Can you work these out from the model? Positions are in its coordinate system, mm. Face numbers are marked on the shaded views. Coordinates: 2 decimals unless noted, no trailing zeros. Loops run counter-clockwise (first coordinate to the right, second up) from the corner with the lowest first, then second, coordinate; pieces in that order, holes last.
```python
from build123d import *

# Parameters (mm, degrees)
F0_W        = 41.65
F0_H        = 46.1
F1_DEPTH    = 6.5
F2_W        = 28.5
F2_H        = 3
F3_DEPTH    = 3
F4_R        = 1
F5_T1_DEPTH = 10.5
F5_T4_ANGLE = 90
F5_T6_ANGLE = 90
F6_W        = 20
F6_H        = 1.8
F7_DEPTH    = 1.8
F8_T1_DEPTH = 21.0093727123
F8_T3_DEPTH = 21.0093727123
F9_SIZE2    = 1.79999
F9_SIZE     = 1.79999
F10_R       = 3


# Not quite as in the source:
# - a fillet or chamfer that OpenCascade refuses, or shapes differently, is made with other operations: its cross-section is extruded or revolved along the edge and cut away or added
# - a fillet or chamfer is up to 0.001 mm smaller than in the source, because OpenCascade refuses the exact size


with BuildPart() as f1:
    # F0 (on Top) → F1 (new body)
    with BuildSketch(Plane.XY):
        Rectangle(F0_W, F0_H)
        with BuildLine():
            ThreePointArc((16.825, -19.85), (17.825, -20.85), (16.825, -21.85))
            Line((16.825, -21.85), (-16.825, -21.85))
            ThreePointArc((-16.825, -21.85), (-17.825, -20.85), (-16.825, -19.85))
            Line((-16.825, -19.85), (16.825, -19.85))
        make_face(mode=Mode.SUBTRACT)
    extrude(amount=F1_DEPTH)

    # F2 (on face) → F3 (join)
    with BuildSketch(Plane(origin=(0, 23.05, 0), x_dir=(-1, 0, 0), z_dir=(0, 1, 0))):
        with Locations((0, 5)):
            Rectangle(F2_W, F2_H)
    extrude(amount=F3_DEPTH)

    # F4
    f4_edges = [f1.edges().sort_by_distance(p)[0] for p in [
        (-14.25, 24.55, 3.5),
        (14.25, 24.55, 3.5),
        (0, 26.05, 3.5),
    ]]
    fillet(f4_edges, radius=F4_R)

    # F5: fillet of radius 3 on 3 edges, made by hand

    # F5_s2 → F5_t1 (cut)
    with BuildSketch(Plane.XY.offset(3.5)):
        with BuildLine():
            ThreePointArc((14.25, 23.05), (13.3713203436, 25.1713203436), (11.25, 26.05))
            Line((11.25, 26.05), (14.25, 26.05))
            Line((14.25, 26.05), (14.25, 23.05))
        make_face()
        with BuildLine():
            ThreePointArc((-14.25, 23.05), (-13.3713203436, 25.1713203436), (-11.25, 26.05))
            Line((-11.25, 26.05), (-14.25, 26.05))
            Line((-14.25, 26.05), (-14.25, 23.05))
        make_face()
    extrude(amount=F5_T1_DEPTH, mode=Mode.SUBTRACT)

    # F5_s3 → F5_t4 (revolve, cut)
    with BuildSketch(Plane.XZ.offset(-23.05)):
        with BuildLine():
            ThreePointArc((-13.25, 3.5), (-13.9571067812, 3.7928932188), (-14.25, 4.5))
            Line((-14.25, 4.5), (-14.25, 3.5))
            Line((-14.25, 3.5), (-13.25, 3.5))
        make_face()
    revolve(axis=Axis((-11.25, 23.05, 3.5), (0, 0, -1)), revolution_arc=F5_T4_ANGLE, mode=Mode.SUBTRACT)

    # F5_s5 → F5_t6 (revolve, cut)
    with BuildSketch(Plane.YZ.offset(11.25)):
        with BuildLine():
            ThreePointArc((25.05, 3.5), (25.7571067812, 3.7928932188), (26.05, 4.5))
            Line((26.05, 4.5), (26.05, 3.5))
            Line((26.05, 3.5), (25.05, 3.5))
        make_face()
    revolve(axis=Axis((11.25, 23.05, 3.5), (0, 0, -1)), revolution_arc=F5_T6_ANGLE, mode=Mode.SUBTRACT)

    # F6 (on face) → F7 (join)
    with BuildSketch(Plane.XZ.offset(23.05)):
        with Locations((0, 4.4)):
            Rectangle(F6_W, F6_H)
        with Locations((0, 0.9)):
            Rectangle(F6_W, F6_H)
    extrude(amount=F7_DEPTH)

    # F8: fillet of radius 5 on 4 edges, made by hand

    # F8_s2 → F8_t1 (cut)
    with BuildSketch(Plane.XY.offset(-6.1046863561)):
        with BuildLine():
            ThreePointArc((-10, -23.05), (-8.2794458011, -24.3776925691), (-6.1581254575, -24.85))
            Line((-6.1581254575, -24.85), (-6.1581254575, -24.95))
            Line((-6.1581254575, -24.95), (-10, -24.95))
            Line((-10, -24.95), (-10.1, -24.85))
            ThreePointArc((-10.1, -24.85), (-10.1, -23.95), (-10.0768374908, -23.114))
            Line((-10.0768374908, -23.114), (-10, -23.05))
        make_face()
        with BuildLine():
            ThreePointArc((10, -23.05), (8.2794458011, -24.3776925691), (6.1581254575, -24.85))
            Line((6.1581254575, -24.85), (6.1581254575, -24.95))
            Line((6.1581254575, -24.95), (10, -24.95))
            Line((10, -24.95), (10.1, -24.85))
            ThreePointArc((10.1, -24.85), (10.1, -23.95), (10.0768374908, -23.114))
            Line((10.0768374908, -23.114), (10, -23.05))
        make_face()
    extrude(amount=F8_T1_DEPTH, mode=Mode.SUBTRACT)

    # F8_s4 → F8_t3 (cut)
    with BuildSketch(Plane.XY.offset(-9.6046863561)):
        with BuildLine():
            ThreePointArc((-10, -23.05), (-8.2794458011, -24.3776925691), (-6.1581254575, -24.85))
            Line((-6.1581254575, -24.85), (-6.1581254575, -24.95))
            Line((-6.1581254575, -24.95), (-10, -24.95))
            Line((-10, -24.95), (-10.1, -24.85))
            ThreePointArc((-10.1, -24.85), (-10.1, -23.95), (-10.0768374908, -23.114))
            Line((-10.0768374908, -23.114), (-10, -23.05))
        make_face()
        with BuildLine():
            ThreePointArc((10, -23.05), (8.2794458011, -24.3776925691), (6.1581254575, -24.85))
            Line((6.1581254575, -24.85), (6.1581254575, -24.95))
            Line((6.1581254575, -24.95), (10, -24.95))
            Line((10, -24.95), (10.1, -24.85))
            ThreePointArc((10.1, -24.85), (10.1, -23.95), (10.0768374908, -23.114))
            Line((10.0768374908, -23.114), (10, -23.05))
        make_face()
    extrude(amount=F8_T3_DEPTH, mode=Mode.SUBTRACT)

    # F9 (size 1.8 and 1.8 in the source; OpenCascade refuses exactly that, so slightly less here)
    f9_edges = [f1.edges().sort_by_distance(p)[0] for p in [
        (0, -24.85, 5.3),
        (0, -24.85, 1.8),
    ]]
    chamfer(f9_edges, length=F9_SIZE, length2=F9_SIZE2)

    # F10
    f10_edges = [f1.edges().sort_by_distance(p)[0] for p in [
        (20.825, -23.05, 3.25),
        (20.825, 23.05, 3.25),
        (-20.825, 23.05, 3.25),
        (-20.825, -23.05, 3.25),
    ]]
    fillet(f10_edges, radius=F10_R)


solid = f1.part
```
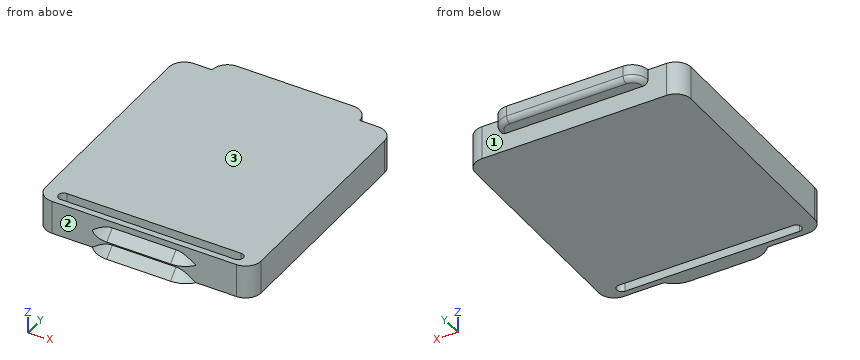
(1) If I drill on probe 1 along Y at (x, z) = (-16.5, 6); probe 2 along Y at (x, z) = (-1.5, 5.75); probe 3 along X at (y, z) = (-21.5, 5.75), over which ranges is the centre line in solid material (lowest first)?
Check values:
probe 1: y = -23.05 to -21.85, -19.85 to 23.05
probe 2: y = -23.05 to -21.85, -19.85 to 26.05
probe 3: x = -20.45 to -17.58, 17.58 to 20.45
(2) I want a section at C-C on z = 1. Write out the boundary of the cut face in (x, y) (3 decimals), then the cut area to 3 significant figures.
Check values:
outline: (-20.825, -20.05) arc R3 ccw to (-17.825, -23.05) - (-8.558, -23.05) arc R4 ccw to (-6.158, -23.85) - (6.158, -23.85) arc R4 ccw to (8.558, -23.05) - (17.825, -23.05) arc R3 ccw to (20.825, -20.05) - (20.825, 20.05) arc R3 ccw to (17.825, 23.05) - (-17.825, 23.05) arc R3 ccw to (-20.825, 20.05) - close; hole (-16.825, -21.85) - (16.825, -21.85) arc R1 ccw to (16.825, -19.85) - (-16.825, -19.85) arc R1 ccw to start
area: 1,850 mm2
(3) I want a section at B-B on y = -20.85. Write out the boundary of the cut face in (x, z) (3 decimals), then the cut area to 3 significant figures.
Check values:
outline: (-20.716, 0) - (-17.825, 0) - (-17.825, 6.5) - (-20.716, 6.5) - close; (17.825, 0) - (20.716, 0) - (20.716, 6.5) - (17.825, 6.5) - close
area: 37.6 mm2
(4) If we mould it in two halves opening along Z, with no side actions, what happens to the marked faces 1, 2 and 3? For each: released by +Z, released by -Z, zero draft, split by the parting line, or undercut.
Check values:
face 1: zero draft
face 2: undercut
face 3: released by +Z
(5) I want a section at D-D on x = 16. Write out the boundary of the cut face in (y, z).
Check values:
outline: (-23.05, 0) - (-21.85, 0) - (-21.85, 6.5) - (-23.05, 6.5) - close; (-19.85, 0) - (23.05, 0) - (23.05, 6.5) - (-19.85, 6.5) - close
(6) I'm going to push flat-ended pins straight in: pin 1 (2 mm diameter, centred on x = -8, z = 5, fed in from -Y); pin 2 (1.6 mm diameter, centred on x = 4.5, y = 24.5, fed in from -Z). Where does each tip first touch, or does it pass through?
Check values:
pin 1: stops at y = -24.03
pin 2: stops at z = 3.5
